Check sheet for the modelled part. Datum: model origin and axes. Units: mm. A direction names the side the tool comes from. Coordinates: 2 decimals unless noted, no trailing zeros. Write each loop counter-clockwise with the first axis right and the second up, starting at its lowest first coordinate (ties: lowest second). Pieces come first, ordered by that corner, then holes. Notation, with made-up numbers: (79.25, 2.5) - (83.25, 2.5) arc R16 cw to (83.25, 25.5) - close; hole circle Ø7 at (48, 48). An arc over 180 degrees is marked (long way). Use one line per item in the form item = value. Start each with the question number.
1. Cross-section at C-C on x = -14. Record the boundary of the cut face in (y, z).
2. Tool access check on faces 4 (the face through (-23.492, -8.005, 32.352)), 5 (the face through (-3.78, -8.07, 3.46)), 6 (the face through (-4, -8, 35.359)). Record the directions out of +Z, -Z, +X, -X, +Y, -Y that give a thin tool (end or side, any length) a straight path to the whole face; none if there is none.
3. Go/stop test with flat-tipped pins: pin 1 Ø3.5 at (x, z) = (-2.46, 3.52) entering from -Y; pin 2 Ø5.5 at (x, y) = (-6.5, -8) entering from +Z; pin 3 Ø10 at (y, z) = (1.5, 24.5) entering from -X; pin 4 Ø8 at (x, y) = (-17, 26.5) entering from -Z. Record where each tip stops, or that it passes through.
4. Scan lines: line 1 along Y through (x, z) = (-20, 18); line 2 along Z through (x, y) = (-4, 12.5); line 3 along Z through (x, y) = (-7, -6). Record each from-to range of solid material in increasing order.
5. Draft check along Y on faces 1 (the face through (-9, -10.54, 17)), 2 (the face through (-8.356, 14.658, 19.77)), 3 (the face through (-7.96, 16.94, 37.4)). Enter one of: +Y half, -Y half, draft (parallel to the pull), parting line (faces both ways), or undercut.
6. Cross-section at A-A on z = 20. Record the boundary of the cut face in (x, y), then the cut area to 3 significant figures.
7. Cross-section at B-B on y = -7. Record the boundary of the cut face in (x, z) (3 decimals), then the cut area to 3 significant figures.
8. Cross-section at D-D on y = -0.5. Give the number of separate pieces and of enclosed holes in the cut face, then the cut area to 3 significant figures.
```python
from build123d import *

# Parameters (mm, degrees)
EXTRUDE_1_DEPTH                  = 40
HOLE_START                       = 0.092539292
HOLE_WIZARD_3_0_2_65_1_OUTLINE_R = 1.325
HOLE_WIZARD_3_0_2_65_1_DEPTH     = 3
SKETCH_7_W                       = 5
SKETCH_7_H                       = 20
CUT_EXTRUDE_1_DEPTH              = 3
HOLE_START_2                     = -10.539590986
HOLE_WIZARD_3_0_2_65_2_OUTLINE_R = 1.325
HOLE_WIZARD_3_0_2_65_2_DEPTH     = 5
HOLE_WIZARD_3_0_2_65_3_OUTLINE_R = 1.325
HOLE_WIZARD_3_0_2_65_3_DEPTH     = 5
FILLET_3_R                       = 2
SKETCH_20_W                      = 36
SKETCH_20_H                      = 4.641244585
CUT_EXTRUDE_3_DEPTH              = 5
SKETCH_23_W                      = 1.741527355
SKETCH_23_H                      = 27.732050807
CUT_EXTRUDE_4_DEPTH              = 3
SKETCH_24_W                      = 1.79143138
SKETCH_24_H                      = 27.732050807
CUT_EXTRUDE_5_DEPTH              = 3
SKETCH_26_W                      = 1.79143138
SKETCH_26_H                      = 1.733650564
EXTRUDE_2_DEPTH                  = 3
FILLET_4_R                       = 10
FILLET_5_R                       = 3
FILLET_6_R                       = 3
FILLET_7_R                       = 3


# Read off the part's stored shape, not the designer's step: Ø3.0 (2.65) 直径孔1, Ø3.0 (2.65) 直径孔2, Ø3.0 (2.65) 直径孔3
with BuildPart() as part:
    # 草图1 → 凸台-拉伸1 (new body)
    with BuildSketch(Plane.XY):
        Polygon((-26.344007522, -10.539590986), (9.655992478, -10.539590986), (-17.096784272, 35.797577588), (-19.694860483, 34.297577588), (3.305139517, -5.539590986), (-26.344007522, -5.539590986), align=None)
    extrude(amount=EXTRUDE_1_DEPTH)

    # Ø3.0 (2.65) 直径孔1 outline → Ø3.0 (2.65) 直径孔1 (cut)
    with BuildSketch(Plane(origin=(0, 0, 0), x_dir=(0.500000000000004, -0.8660254037844363, 0), z_dir=(0.8660254037844363, 0.5000000000000042, 0)).offset(HOLE_START)):
        with Locations((1.719905554, -5.253562617)):
            Circle(HOLE_WIZARD_3_0_2_65_1_OUTLINE_R)
        with Locations((1.719905554, -34.903562617)):
            Circle(HOLE_WIZARD_3_0_2_65_1_OUTLINE_R)
    extrude(amount=HOLE_WIZARD_3_0_2_65_1_DEPTH, mode=Mode.SUBTRACT)

    # 草图7 → 切除-拉伸1 (cut)
    with BuildSketch(Plane(origin=(2.678217589, 1.546269646, 0), x_dir=(0, 0, -1), z_dir=(0.8660254037844364, 0.5000000000000041, 0))):
        with Locations((-37.5, 29.550003721)):
            Rectangle(SKETCH_7_W, SKETCH_7_H)
        with Locations((-2.5, 29.550003721)):
            Rectangle(SKETCH_7_W, SKETCH_7_H)
    extrude(amount=-CUT_EXTRUDE_1_DEPTH, mode=Mode.SUBTRACT)

    # Ø3.0 (2.65) 直径孔2 outline → Ø3.0 (2.65) 直径孔2 (cut)
    with BuildSketch(Plane(origin=(0, 0, 0), x_dir=(1, 0, 0), z_dir=(0, 1, 0)).offset(HOLE_START_2)):
        with Locations((-9.458240247, -3.522342215)):
            Circle(HOLE_WIZARD_3_0_2_65_2_OUTLINE_R)
        with Locations((-2.458240247, -3.522342215)):
            Circle(HOLE_WIZARD_3_0_2_65_2_OUTLINE_R)
    extrude(amount=HOLE_WIZARD_3_0_2_65_2_DEPTH, mode=Mode.SUBTRACT)

    # Ø3.0 (2.65) 直径孔3 outline → Ø3.0 (2.65) 直径孔3 (cut)
    with BuildSketch(Plane(origin=(0, 0, 0), x_dir=(1, 0, 0), z_dir=(0, 1, 0)).offset(HOLE_START_2)):
        with Locations((-1.947010607, -36.908916004)):
            Circle(HOLE_WIZARD_3_0_2_65_3_OUTLINE_R)
        with Locations((-8.947010607, -36.908916004)):
            Circle(HOLE_WIZARD_3_0_2_65_3_OUTLINE_R)
    extrude(amount=HOLE_WIZARD_3_0_2_65_3_DEPTH, mode=Mode.SUBTRACT)

    # 圆角3
    fillet_3_edges = [part.edges().sort_by_distance(p)[0] for p in [
        (-18.395822378, 35.047577588, 35),
        (-18.395822378, 35.047577588, 5),
    ]]
    fillet(fillet_3_edges, radius=FILLET_3_R)

    # 草图20 → 切除-拉伸3 (cut)
    with BuildSketch(Plane.XZ.offset(10.539590986)):
        with Locations((-8.344007522, 37.679377708)):
            Rectangle(SKETCH_20_W, SKETCH_20_H)
    extrude(amount=-CUT_EXTRUDE_3_DEPTH, mode=Mode.SUBTRACT)

    # 草图23 → 切除-拉伸4 (cut)
    with BuildSketch(Plane(origin=(2.678217589, 1.546269646, 0), x_dir=(0, 0, -1), z_dir=(0.8660254037844364, 0.5000000000000041, 0))):
        with Locations((-39.129236323, 5.683978317)):
            Rectangle(SKETCH_23_W, SKETCH_23_H)
    extrude(amount=-CUT_EXTRUDE_4_DEPTH, mode=Mode.SUBTRACT)

    # 草图24 → 切除-拉伸5 (cut)
    with BuildSketch(Plane(origin=(2.678217589, 1.546269646, 0), x_dir=(0, 0, -1), z_dir=(0.8660254037844364, 0.5000000000000041, 0))):
        with Locations((-0.89571569, 5.683978317)):
            Rectangle(SKETCH_24_W, SKETCH_24_H)
    extrude(amount=-CUT_EXTRUDE_5_DEPTH, mode=Mode.SUBTRACT)

    # 草图26 → 凸台-拉伸2 (add)
    with BuildSketch(Plane(origin=(0.080141377, 0.046269646, 0), x_dir=(0, 0, -1), z_dir=(0.8660254037844364, 0.5000000000000041, 0))):
        with Locations((-0.89571569, -7.316821561)):
            Rectangle(SKETCH_26_W, SKETCH_26_H)
    extrude(amount=EXTRUDE_2_DEPTH)

    # 圆角4
    fillet_4_edges = [part.edges().sort_by_distance(p)[0] for p in [
        (-26.344007522, -8.039590986, 35.358755415),
        (-26.344007522, -8.039590986, 0),
    ]]
    fillet(fillet_4_edges, radius=FILLET_4_R)

    # 圆角5
    fillet_5_edges = [part.edges().sort_by_distance(p)[0] for p in [
        (-8.395822378, 17.727069512, 38.258472645),
        (-8.395822378, 17.727069512, 1.79143138),
    ]]
    fillet(fillet_5_edges, radius=FILLET_5_R)

    # 圆角6
    # the kernel refuses this fillet: 3 mm, written as the material it takes off along each edge
    with BuildSketch(Plane(origin=(14.265049697, -5.539590986, 38.258472645), x_dir=(0, 0, -1), z_dir=(-1, 0, 0))) as fillet_6_piece_1:
        with BuildLine():
            CenterArc((3, -2.998323426), FILLET_6_R, 91.915616688, 88.084383312)
            Line((0, -2.998323426), (-0.06, -2.998323426))
            Line((-0.06, -2.998323426), (-0.06, 0))
            Line((-0.06, 0), (0, 0.06))
            ThreePointArc((0, 0.06), (1.449858615, 0.06), (2.897711575, 0.059966469))
            Line((2.897711575, 0.059966469), (2.89971723, 0))
        make_face()
    extrude(amount=18.455718744, mode=Mode.SUBTRACT)

    # 圆角7
    # the kernel refuses this fillet: 3 mm, written as the material it takes off along each edge
    with BuildSketch(Plane(origin=(-2.639669888, -8.971828296, 0), x_dir=(0, 0, 1), z_dir=(0.8660254037844363, 0.5000000000000041, 0))) as fillet_7_piece_1_section:
        with BuildLine():
            CenterArc((3, 2.745789848), FILLET_7_R, 180, 66.243144393)
            Line((0, 2.745789848), (0, 0))
            Line((0, 0), (1.79143138, 0))
        make_face()
    fillet_7_piece_1 = extrude(amount=16.728949241, mode=Mode.PRIVATE)
    fillet_7_piece_1 = split(fillet_7_piece_1, bisect_by=Plane(origin=(4.952096939, -5.539590986, 0.801424093), z_dir=(0, 1, 0)), keep=Keep.TOP, mode=Mode.PRIVATE)
    add(fillet_7_piece_1, mode=Mode.SUBTRACT)


solid = part.part
```
Final values:
q1.outline = (-10.54, 0) - (-5.54, 0) - (-5.54, 35.36) - (-10.54, 35.36) - close; (24.43, 5) - (30.43, 5) - (30.43, 35) - (24.43, 35) - close
q2.face_4 = +Z, -X, +Y, -Y
q2.face_5 = -Y
q2.face_6 = +Z, +X, -X, -Y
q3.pin_1 = -10.54
q3.pin_2 = 35.36
q3.pin_3 = -3.65
q3.pin_4 = 5
q4.line_1 = -10.54 to -5.54
q4.line_2 = 1.79 to 38.26
q4.line_3 = 0 to 35.36
q5.face_1 = -Y half
q5.face_2 = undercut
q5.face_3 = +Y half
q6.outline = (-26.34, -10.54) - (9.66, -10.54) - (-17.1, 35.8) - (-19.69, 34.3) - (3.31, -5.54) - (-26.34, -5.54) - close
q6.area = 313 mm²
q7.outline = (-26.344, 10) arc R10 ccw to (-16.344, 0) - (7.612, 0) - (7.612, 35.359) - (-16.344, 35.359) arc R10 ccw to (-26.344, 25.359) - close; hole circle Ø2.65 at (-9.458, 3.522); hole circle Ø2.65 at (-2.458, 3.522)
q7.area = 1,150 mm²
q8.separate_pieces = 3
q8.enclosed_holes = 0
q8.area = 110 mm²
